Verification items for the finished model (mm, model axes). A direction names the side the tool comes from. Round coordinates to 2 decimals unless told otherwise and drop trailing zeros. Write each loop counter-clockwise with the first axis right and the second up, starting at its lowest first coordinate (ties: lowest second). Pieces come first, ordered by that corner, then holes. Notation, with made-up numbers: M -16.5,-4.5 L 38.5,-4.5 A15 cw 38.5,19.5 Z; hole C 65.25,-8 d3. An arc over 180 degrees is marked long. One line per question, with ' | ' between items.
from build123d import *

# Parameters (mm, degrees)
EXTRUDE_1_DEPTH     = 5
SKETCH_3_R          = 2.5
CUT_EXTRUDE_1_DEPTH = 24
SKETCH_4_R          = 1.525
CUT_EXTRUDE_2_DEPTH = 5
SKETCH_5_R          = 2.5
CUT_EXTRUDE_3_DEPTH = 5
FILLET_1_R          = 5


with BuildPart() as part:
    # 草图1 → 凸台-拉伸1 (new body)
    with BuildSketch(Plane.XY):
        with BuildLine():
            Line((5, -8.077747211), (5, -45))
            ThreePointArc((5, -45), (0, -50), (-5, -45))
            Line((-5, -45), (-5, -8.077747211))
            ThreePointArc((-5, -8.077747211), (0, 9.5), (5, -8.077747211))
        make_face()
    extrude(amount=EXTRUDE_1_DEPTH)

    # 草图3 → 切除-拉伸1 (cut)
    with BuildSketch(Plane.XY.offset(5)):
        with Locations((0, -45)):
            Circle(SKETCH_3_R)
    extrude(amount=-CUT_EXTRUDE_1_DEPTH, mode=Mode.SUBTRACT)

    # 草图4 → 切除-拉伸2 (cut)
    with BuildSketch(Plane.XY.offset(5)):
        with Locations((0, 6.25)):
            Circle(SKETCH_4_R)
        with Locations((0, -6.25)):
            Circle(SKETCH_4_R)
    extrude(amount=-CUT_EXTRUDE_2_DEPTH, mode=Mode.SUBTRACT)

    # 草图5 → 切除-拉伸3 (cut)
    with BuildSketch(Plane.XY.offset(5)):
        Circle(SKETCH_5_R)
    extrude(amount=-CUT_EXTRUDE_3_DEPTH, mode=Mode.SUBTRACT)

    # 圆角1
    fillet_1_edges = [part.edges().sort_by_distance(p)[0] for p in [
        (-5, -8.077747211, 2.5),
        (5, -8.077747211, 2.5),
    ]]
    fillet(fillet_1_edges, radius=FILLET_1_R)


solid = part.part
1. Section check A-A, the plane y = 0. Record the cut outline in (x, z).
Results:
outline: M -9.5,0 L -2.5,0 L -2.5,5 L -9.5,5 Z; M 2.5,0 L 9.5,0 L 9.5,5 L 2.5,5 Z
2. Mould release check, pull along Y, two halves, no side actions. Record for faces 3 (the face through (-0.317, 9.495, 2.465)), 4 (the face through (0, -50, 2)), 5 (the face through (-5, -28, 2)), 6 (the face through (0.82, 7.536, 2.535)): pulls with the +Y half, pulls with the -Y half, needs draft (parallel to the pull), parting line crosses it, or undercut.
Results:
face 3: parting line crosses it | face 4: pulls with the -Y half | face 5: needs draft | face 6: undercut
3. Section check C-C, the plane z = 3.5. Record the cut outline in (x, y) (3 decimals).
Results:
outline: M -6.552,-6.879 A5 cw -5,-10.5 L -5,-45 A5 ccw 5,-45 L 5,-10.5 A5 cw 6.552,-6.879 A9.5 ccw long Z; hole C 0,-45 d5; hole C 0,0 d5; hole C 0,-6.25 d3.05; hole C 0,6.25 d3.05
4. Tool access check on faces 1 (the face through (0, -20, 5)), 2 (the face through (5, -28, 2)). Record the directions out of +Z, -Z, +X, -X, +Y, -Y that give a thin tool (end or side, any length) a straight path to the whole face; none if there is none.
Results:
face 1: +Z, +X, -X, +Y, -Y | face 2: +Z, -Z, +X, -Y
5. Go/stop test with flat-tipped pins: P1, Ø1, axis at x = -3.5, z = 3, coming from the -Y side; P2, Ø3, axis at x = -4, y = 2, coming from the -Z side; P3, Ø1.5, axis at y = -30, z = 1.5, coming from the -X side. Record where each tip stops, or that it passes through.
Results:
P1: stops at y = -49 | P2: stops at z = 0 | P3: stops at x = -5
6. Section check B-B, the plane x = 0. Record the cut outline in (y, z) (3 decimals).
Results:
outline: M -50,0 L -47.5,0 L -47.5,5 L -50,5 Z; M -42.5,0 L -7.775,0 L -7.775,5 L -42.5,5 Z; M -4.725,0 L -2.5,0 L -2.5,5 L -4.725,5 Z; M 2.5,0 L 4.725,0 L 4.725,5 L 2.5,5 Z; M 7.775,0 L 9.5,0 L 9.5,5 L 7.775,5 Z
7. Thickness scan on line 1 (Y direction, x = 0, z = 1.55) (3 decimals); line 2 (X direction, y = -26.5, z = 3.35); line 3 (Y direction, x = 2, z = 0.45). Record the ranges inside material, lowest first.
Results:
line 1: y = -50 to -47.5, -42.5 to -7.775, -4.725 to -2.5, 2.5 to 4.725, 7.775 to 9.5 | line 2: x = -5 to 5 | line 3: y = -49.58 to -46.5, -43.5 to -1.5, 1.5 to 9.29
8. Section check D-D, the plane y = 6.25. Record the cut outline in (x, z) (3 decimals).
Results:
outline: M -7.155,0 L -1.525,0 L -1.525,5 L -7.155,5 Z; M 1.525,0 L 7.155,0 L 7.155,5 L 1.525,5 Z
